For this review, take the finished solid that the model builds, in its own axes (mm). A direction names the side the tool comes from. Give positions to 0.01 mm unless a question says otherwise; leave off trailing zeros. Order: outer loops, then holes, each group sorted by start corner. A loop starts at its lowest first (then second) coordinate and runs counter-clockwise, first axis right, second up. Notation, with made-up numbers: (9, 73.5) - (27, 73.5) arc R12 ccw to (27, 94.5) - close; hole circle Ø3 at (46.25, 67). An arc over 180 degrees is marked (long way). One line per item, written item: value.
```python
from build123d import *

# Parameters (mm, degrees)
SKETCH1_R                                       = 10
BOSS_EXTRUDE1_DEPTH                             = 40
SKETCH2_R                                       = 14
CUT_EXTRUDE1_DEPTH                              = 12
CUT_EXTRUDE2_START                              = -10
SKETCH3_R                                       = 14
CUT_EXTRUDE2_DEPTH                              = 10
SKETCH5_R                                       = 19.05
CUT_EXTRUDE3_DEPTH                              = 2
CBORE_FOR_M5_HEX_HEAD_BOLT1_D                   = 5.5
CBORE_FOR_M5_HEX_HEAD_BOLT1_CBORE_D             = 12.24
CBORE_FOR_M5_HEX_HEAD_BOLT1_CBORE_DEPTH         = 8.58
CSK_FOR_M4_FLAT_HEAD_MACHINE_SCREW1_D           = 4.5
CSK_FOR_M4_FLAT_HEAD_MACHINE_SCREW1_CSINK_D     = 9.4
CSK_FOR_M4_FLAT_HEAD_MACHINE_SCREW1_CSINK_ANGLE = 90
LPATTERN1_COUNT                                 = 2
LPATTERN1_PITCH                                 = 23
LPATTERN1_COUNT_DIR2                            = 2
LPATTERN1_PITCH_DIR2                            = 70
SKETCH13_R                                      = 7.5
CUT_EXTRUDE4_DEPTH                              = 136.576546644
SKETCH14_R                                      = 20.000672508
CUT_EXTRUDE5_DEPTH                              = 136.576546644


with BuildPart() as part:
    # Sketch1 → Boss-Extrude1 (new body)
    with BuildSketch(Plane(origin=(0, 0, 0), x_dir=(1, 0, 0), z_dir=(0, 1, 0))):
        Polygon((0, 0), (-10, 0), (-10, -6), (70, -6), (70, 0), (60, 0), (60, 109), (0, 109), align=None)
        with Locations(Location((30, 74, 0), (0, 0, 270))):
            Circle(SKETCH1_R, mode=Mode.SUBTRACT)
    extrude(amount=BOSS_EXTRUDE1_DEPTH)

    # Sketch2 → Cut-Extrude1 (cut)
    with BuildSketch(Plane.XZ):
        with Locations(Location((30, -74, 0), (0, 0, 270))):
            Circle(SKETCH2_R)
    extrude(amount=-CUT_EXTRUDE1_DEPTH, mode=Mode.SUBTRACT)

    # Sketch3 → Cut-Extrude2 (cut)
    with BuildSketch(Plane(origin=(0, 40, 0), x_dir=(1, 0, 0), z_dir=(0, 1, 0)).offset(CUT_EXTRUDE2_START)):
        with Locations(Location((30, 74, 0), (0, 0, 90))):
            Circle(SKETCH3_R)
    extrude(amount=CUT_EXTRUDE2_DEPTH, mode=Mode.SUBTRACT)

    # Sketch5 → Cut-Extrude3 (cut)
    with BuildSketch(Plane.XZ):
        with Locations(Location((30, -74, 0), (0, 0, 270))):
            Circle(SKETCH5_R)
    extrude(amount=-CUT_EXTRUDE3_DEPTH, mode=Mode.SUBTRACT)

    # CBORE for M5 Hex Head Bolt1 (through all)
    with Locations(Plane(origin=(0, 40, 0), x_dir=(-1, 0, 0), z_dir=(0, 1, 0))):
        with Locations((-6.43, -97.57), (-6.43, -50.43), (-53.57, -50.43), (-53.57, -97.57)):
            CounterBoreHole(CBORE_FOR_M5_HEX_HEAD_BOLT1_D / 2, CBORE_FOR_M5_HEX_HEAD_BOLT1_CBORE_D / 2, CBORE_FOR_M5_HEX_HEAD_BOLT1_CBORE_DEPTH)

    # CSK for M4 Flat Head Machine Screw1 (through all)
    with Locations(Plane(origin=(0, 0, 0), x_dir=(-1, 0, 0), z_dir=(0, 0, -1))):
        with Locations((-65, 6)):
            csk_for_m4_flat_head_machine_screw1 = CounterSinkHole(CSK_FOR_M4_FLAT_HEAD_MACHINE_SCREW1_D / 2, CSK_FOR_M4_FLAT_HEAD_MACHINE_SCREW1_CSINK_D / 2, counter_sink_angle=CSK_FOR_M4_FLAT_HEAD_MACHINE_SCREW1_CSINK_ANGLE)

    # LPattern1: CSK for M4 Flat Head Machine Screw1 2 × 2
    with Locations(*[(-j * LPATTERN1_PITCH_DIR2, i * LPATTERN1_PITCH, 0) for i in range(LPATTERN1_COUNT) for j in range(LPATTERN1_COUNT_DIR2) if (i, j) != (0, 0)]):
        add(csk_for_m4_flat_head_machine_screw1, mode=Mode.SUBTRACT)

    # Sketch13 → Cut-Extrude4 (cut, through all)
    with BuildSketch(Plane(origin=(60, 0, 0), x_dir=(0, 0, -1), z_dir=(1, 0, 0))):
        with Locations((74, 20)):
            Circle(SKETCH13_R)
    extrude(amount=-CUT_EXTRUDE4_DEPTH, mode=Mode.SUBTRACT)

    # Sketch14 → Cut-Extrude5 (cut, through all)
    with BuildSketch(Plane.XZ):
        with Locations(Location((30, -24, 0), (0, 0, 270))):
            Circle(SKETCH14_R)
    extrude(amount=-CUT_EXTRUDE5_DEPTH, mode=Mode.SUBTRACT)


solid = part.part
```
(1) Take a section at B-B (z = -24). Write out the cut boundary in (x, y).
Answers below:
outline: (0, 0) - (10, 0) - (10, 40) - (0, 40) - close; (50, 0) - (60, 0) - (60, 40) - (50, 40) - close
(2) Take a section at C-C (x = 53.57). Write out the cut boundary in (y, z), then the cut area to 3 significant figures.
Answers below:
outline: (0, -109) - (40, -109) - (40, -103.69) - (31.42, -103.69) - (31.42, -100.32) - (0, -100.32) - close; (0, -94.82) - (31.42, -94.82) - (31.42, -91.45) - (40, -91.45) - (40, -56.55) - (31.42, -56.55) - (31.42, -53.18) - (0, -53.18) - close; (0, -47.68) - (31.42, -47.68) - (31.42, -44.31) - (40, -44.31) - (40, 6) - (0, 6) - close; hole circle Ø15 at (20, -74)
area: 3,870 mm^2
(3) Take a section at A-A (y = 6). Give the number of separate pieces and of enclosed holes in the cut face, then the cut area to 3 significant figures.
Answers below:
separate pieces: 3
enclosed holes: 6
area: 4,990 mm^2
(4) Machinability: for faces 5 (the face through (65, 20, 0)), 6 (the face through (11.29, 35.77, -101.29)), 7 (the face through (40, 12, -71)), which of the approach directions +Z, -Z, +X, -X, +Y, -Y give a long, thin tool a straight path to every point of the face, cutting with its end or side? Answer none if there is none.
Answers below:
face 5: -Z, +X, +Y, -Y
face 6: +Y
face 7: -Y
(5) Take a section at D-D (z = -50.43). Write out the cut boundary in (x, y).
Answers below:
outline: (0, 0) - (3.68, 0) - (3.68, 31.42) - (0.31, 31.42) - (0.31, 40) - (0, 40) - close; (9.18, 0) - (50.82, 0) - (50.82, 31.42) - (47.45, 31.42) - (47.45, 40) - (12.55, 40) - (12.55, 31.42) - (9.18, 31.42) - close; (56.32, 0) - (60, 0) - (60, 40) - (59.69, 40) - (59.69, 31.42) - (56.32, 31.42) - close
(6) Draft analysis for pull direction X (two halves, no side actions). For faces 1 (the face through (48.47, 12.68, -72.37)), 2 (the face through (0, 20, -55)), 3 (the face through (70, 20, 3)), 4 (the face through (7.757, 35.77, -56.404)), state which applies: pulls with the +X half, pulls with the -X half, needs draft (parallel to the pull), parting line crosses it, or undercut.
Answers below:
face 1: needs draft
face 2: pulls with the -X half
face 3: pulls with the +X half
face 4: undercut
(7) Wall thickness on line 1 (Y direction, x = 47, z = -74); line 2 (X direction, y = 34, z = -96.5); line 3 (Z direction, x = 12.5, y = 18.5): over which ranges is each line inside the solid? List them lowest first. Write a range as from..to.
Answers below:
line 1: y = 2..12.5, 27.5..40
line 2: x = 0..0.4, 12.46..47.54, 59.6..60
line 3: z = -109..-81.35, -66.65..-33.68, -14.32..6
(8) For P1, Ø4, axis at y = 34, z = -34.5, coming from the -X side; P2, Ø6, axis at y = 26.5, z = -36.5, coming from the +X side; P3, Ø3.5, axis at x = 52.5, z = -95.5, coming from the +Y side, all flat-tipped, find the tip position at first contact; note any pin that passes through.
Answers below:
P1: stops at x = 0
P2: stops at x = 60
P3: stops at y = 31.42
